Source: CAD feature listing. Evaluate the final solid. Frame: model axes, mm. Give positions to 0.01 mm unless a question says otherwise; leave off trailing zeros. Order: outer loops, then holes, each group sorted by start corner. A loop starts at its lowest first (then second) coordinate and runs counter-clockwise, first axis right, second up.
1) First-contact query: P1, Ø1.9, axis at x = 157.5, y = 7.5, coming from the -Z side; P2, Ø4, axis at x = 485, z = 7.5, coming from the -Y side. Flat tips, straight axial feed; report the tip coordinate or a pass-through.
2) Section A-A, the plane y = 3.5. Return loops of the section in (x, z), plus the area to 3 significant figures.
3) Material intervals for line 1 (Z direction, x = 158.5, y = 3.25); line 2 (Y direction, x = 307.5, z = 14.3), sorted ascending.
4) Section B-B, the plane x = 439. Return loops of the section in (y, z).
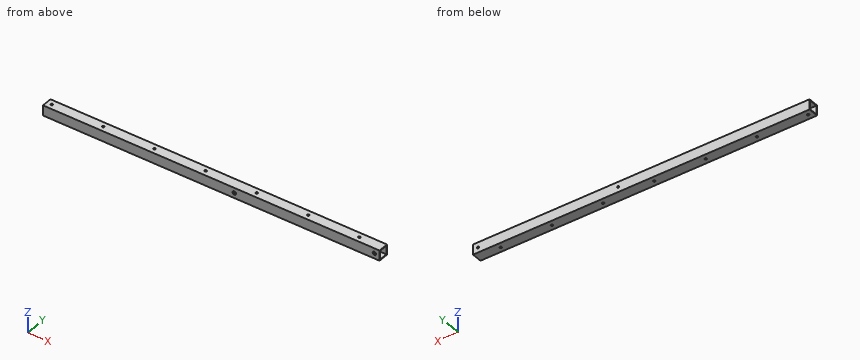
```python
from build123d import *

# Parameters (mm, degrees)
SKETCH_2_W          = 492.5
SKETCH_2_H          = 15
SKETCH_2_R          = 1.6
EXTRUDE_1_DEPTH     = 15
SKETCH_3_W          = 12.6
SKETCH_3_H          = 12.6
CUT_EXTRUDE_1_DEPTH = 493.956641095
SKETCH_4_R          = 1.5
CUT_EXTRUDE_2_DEPTH = 493.956641095
CHAMFER_1_SIZE      = 1


with BuildPart() as part:
    # ｽｹｯﾁ2 → ﾎﾞｽ - 押し出し1 (new body)
    with BuildSketch(Plane.XY):
        with Locations((246.25, 7.5)):
            Rectangle(SKETCH_2_W, SKETCH_2_H)
        with Locations((7.5, 7.5)):
            Circle(SKETCH_2_R, mode=Mode.SUBTRACT)
        with Locations((457.5, 7.5)):
            Circle(SKETCH_2_R, mode=Mode.SUBTRACT)
        with Locations((232.5, 7.5)):
            Circle(SKETCH_2_R, mode=Mode.SUBTRACT)
        with Locations((82.5, 7.5)):
            Circle(SKETCH_2_R, mode=Mode.SUBTRACT)
        with Locations((157.5, 7.5)):
            Circle(SKETCH_2_R, mode=Mode.SUBTRACT)
        with Locations((307.5, 7.5)):
            Circle(SKETCH_2_R, mode=Mode.SUBTRACT)
        with Locations((382.5, 7.5)):
            Circle(SKETCH_2_R, mode=Mode.SUBTRACT)
    extrude(amount=EXTRUDE_1_DEPTH)

    # ｽｹｯﾁ3 → ｶｯﾄ - 押し出し1 (cut, through all)
    with BuildSketch(Plane(origin=(492.5, 0, 0), x_dir=(0, 0, -1), z_dir=(1, 0, 0))):
        with Locations((-7.5, 7.5)):
            Rectangle(SKETCH_3_W, SKETCH_3_H)
    extrude(amount=-CUT_EXTRUDE_1_DEPTH, mode=Mode.SUBTRACT)

    # ｽｹｯﾁ4 → ｶｯﾄ - 押し出し2 (cut, through all)
    with BuildSketch(Plane(origin=(0, 15, 0), x_dir=(1, 0, 0), z_dir=(0, 1, 0))):
        with Locations(Location((280, -7.5, 0), (0, 0, 180))):
            Circle(SKETCH_4_R)
        with Locations(Location((485, -7.5, 0), (0, 0, 180))):
            Circle(SKETCH_4_R)
    extrude(amount=-CUT_EXTRUDE_2_DEPTH, mode=Mode.SUBTRACT)

    # 面取り1
    chamfer_1_edges = [part.edges().sort_by_distance(p)[0] for p in [
        (281.5, 0, 7.5),
        (486.5, 0, 7.5),
    ]]
    chamfer(chamfer_1_edges, length=CHAMFER_1_SIZE)


solid = part.part
```
From the geometry:
1. P1: passes through
1. P2: stops at y = 0.5
2. outline: (0, 0) - (492.5, 0) - (492.5, 1.2) - (0, 1.2) - close; (0, 13.8) - (492.5, 13.8) - (492.5, 15) - (0, 15) - close
2. area: 1,180 mm2
3. line 1: z = 0 to 1.2, 13.8 to 15
3. line 2: y = 0 to 5.9, 9.1 to 15
4. outline: (0, 0) - (15, 0) - (15, 15) - (0, 15) - close; hole (1.2, 1.2) - (13.8, 1.2) - (13.8, 13.8) - (1.2, 13.8) - close
